The figure shows three views and two pictorial views of one solid part (mm, origin at its lowest corner). Answer the questions. Round coordinates to 2 decimals unless told otherwise and drop trailing zeros. Order: outer loops, then holes, each group sorted by start corner. A loop starts at its lowest first (then second) coordinate and runs counter-clockwise, first axis right, second up. Notation, with made-up numbers: (-33.5, -12.75) -> (-8.5, -12.75) arc R22 cw to (-8.5, 11.25) -> close; hole circle Ø7 at (-6.75, 2.25). An arc over 180 degrees is marked (long way). Return JSON: item names as keys, results as strings. Group by question number.
(1) Each of these flat-tipped pins is pushed along its axis until it touches: pin 1 (3.5 mm diameter, centred on y = 61, z = 8, fed in from +X); pin 2 (6 mm diameter, centred on x = 61.5, z = 9.5, fed in from +Y); pin 3 (1.5 mm diameter, centred on x = 89, z = 12, fed in from +Y). Where does it stop, or does it pass through?
(2) The part is cut by section B-B (y = 50). Determine the outline of the cut face in (x, z).
(3) The part is cut by section A-A (x = 50). Determine the outline of the cut face in (y, z).
(4) Determine the mould class of the marked faces 1, 2, 3 and 4 for opening direction Y: +Y half, -Y half, draft (parallel to the pull), parting line (faces both ways), or undercut.
(5) The part is cut by section C-C (z = 23.25). Determine the outline of the cut face in (x, y).
(6) Consider line 1 (Y direction, x = 50, z = 16); line 2 (X direction, y = 46, z = 12.5); line 3 (X direction, y = 23, z = 9.25). Determine where each line is inside the solid, lowest interval first. Write a range as [from, to].
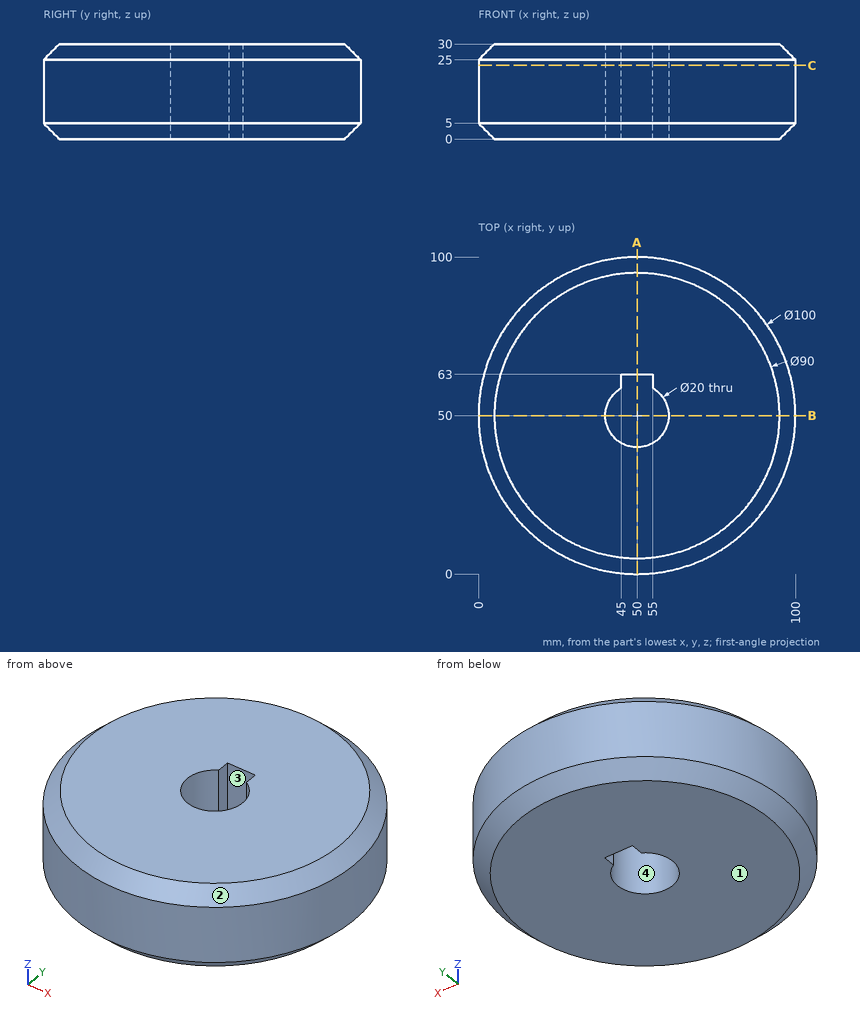
Answer below:
{
 "1": {"pin 1": "stops at x = 99.14", "pin 2": "stops at y = 99.27", "pin 3": "stops at y = 82.2"},
 "2": {"outline": "(0, 5) -> (5, 0) -> (40, 0) -> (40, 30) -> (5, 30) -> (0, 25) -> close; (60, 0) -> (95, 0) -> (100, 5) -> (100, 25) -> (95, 30) -> (60, 30) -> close"},
 "3": {"outline": "(0, 5) -> (5, 0) -> (40, 0) -> (40, 30) -> (5, 30) -> (0, 25) -> close; (63, 0) -> (95, 0) -> (100, 5) -> (100, 25) -> (95, 30) -> (63, 30) -> close"},
 "4": {"face 1": "draft", "face 2": "parting line", "face 3": "undercut", "face 4": "undercut"},
 "5": {"outline": "circle Ø100 at (50, 50); hole (45, 58.66) arc R10 ccw (long way) to (55, 58.66) -> (55, 63) -> (45, 63) -> close"},
 "6": {"line 1": "y = [0, 40], [63, 100]", "line 2": "x = [0.16, 40.83], [59.17, 99.84]", "line 3": "x = [7.92, 92.08]"}
}
